from build123d import *

# Parameters (mm, degrees)
SKETCH1_R           = 50.8
BOSS_EXTRUDE1_DEPTH = 25
FILLET2_R           = 8
FILLET3_R           = 8
SKETCH2_R           = 15
BOSS_EXTRUDE2_DEPTH = 5
SKETCH3_R           = 12
CUT_EXTRUDE1_DEPTH  = 5
FILLET4_R           = 8
SKETCH5_R           = 3.165
CUT_EXTRUDE2_DEPTH  = 78.85422275
CUT_EXTRUDE3_DEPTH  = 78.85422275


with BuildPart() as part:
    # Sketch1 → Boss-Extrude1 (new body)
    with BuildSketch(Plane(origin=(0, 0, 0), x_dir=(1, 0, 0), z_dir=(0, 1, 0))):
        with Locations(Location((0, 0, 0), (0, 0, 270))):
            Circle(SKETCH1_R)
    extrude(amount=BOSS_EXTRUDE1_DEPTH)

    # Fillet2
    fillet2_edges = [part.edges().sort_by_distance(p)[0] for p in [
        (0, 25, -50.8),
    ]]
    fillet(fillet2_edges, radius=FILLET2_R)

    # Fillet3
    fillet3_edges = [part.edges().sort_by_distance(p)[0] for p in [
        (0, 0, -50.8),
    ]]
    fillet(fillet3_edges, radius=FILLET3_R)

    # Sketch2 → Boss-Extrude2 (add)
    with BuildSketch(Plane.XZ):
        with Locations(Location((0, 0, 0), (0, 0, 90))):
            Circle(SKETCH2_R)
    extrude(amount=BOSS_EXTRUDE2_DEPTH)

    # Sketch3 → Cut-Extrude1 (cut)
    with BuildSketch(Plane(origin=(0, 25, 0), x_dir=(1, 0, 0), z_dir=(0, 1, 0))):
        with Locations(Location((0, 0, 0), (0, 0, 270))):
            Circle(SKETCH3_R)
    extrude(amount=-CUT_EXTRUDE1_DEPTH, mode=Mode.SUBTRACT)

    # Fillet4
    # the kernel refuses this fillet: 8 mm, written as the material it adds along each edge
    with BuildSketch(Plane(origin=(0, 0, 0), x_dir=(0, 0, 1), z_dir=(1, 0, 0))) as fillet4_piece_1:
        with BuildLine():
            CenterArc((22.416198487, 8), FILLET4_R, 202.024312837, 67.975687163)
            Line((15, 5), (14.85167603, 4.94))
            ThreePointArc((14.85167603, 4.94), (14.84, 2.5), (14.84, 0))
            Line((14.84, 0), (15, -0.16))
            Line((15, -0.16), (22.416198487, -0.16))
            Line((22.416198487, -0.16), (22.416198487, 0))
        make_face()
    revolve(axis=Axis((0, 0, 0), (0, -1, 0)))

    # Sketch5 → Cut-Extrude2 (cut, through all)
    with BuildSketch(Plane.XZ.offset(5)):
        with Locations(Location((0, 0, 0), (0, 0, 270))):
            Circle(SKETCH5_R)
    extrude(amount=-CUT_EXTRUDE2_DEPTH, mode=Mode.SUBTRACT)

    # Sketch6 → Cut-Extrude3 (cut, through all)
    with BuildSketch(Plane(origin=(0, 25, 0), x_dir=(1, 0, 0), z_dir=(0, 1, 0))):
        with BuildLine():
            Line((6.669640143, 14.619160774), (17.119775233, 37.524775128))
            ThreePointArc((17.119775233, 37.524775128), (-2.42176691, 41.174391282), (-21.4007271, 35.259102825))
            Line((-21.4007271, 35.259102825), (-8.337442905, 13.736484528))
            ThreePointArc((-8.337442905, 13.736484528), (-0.943488661, 16.041003414), (6.669640143, 14.619160774))
        make_face()
        with BuildLine():
            Line((13.736484528, 8.337442905), (35.259102825, 21.4007271))
            ThreePointArc((35.259102825, 21.4007271), (41.174391282, 2.42176691), (37.524775128, -17.119775233))
            Line((37.524775128, -17.119775233), (14.619160774, -6.669640143))
            ThreePointArc((14.619160774, -6.669640143), (16.041003414, 0.943488661), (13.736484528, 8.337442905))
        make_face()
        with BuildLine():
            Line((8.337442905, -13.736484528), (21.4007271, -35.259102825))
            ThreePointArc((21.4007271, -35.259102825), (2.42176691, -41.174391282), (-17.119775233, -37.524775128))
            Line((-17.119775233, -37.524775128), (-6.669640143, -14.619160774))
            ThreePointArc((-6.669640143, -14.619160774), (0.943488661, -16.041003414), (8.337442905, -13.736484528))
        make_face()
        with BuildLine():
            Line((-13.736484528, -8.337442905), (-35.259102825, -21.4007271))
            ThreePointArc((-35.259102825, -21.4007271), (-41.174391282, -2.42176691), (-37.524775128, 17.119775233))
            Line((-37.524775128, 17.119775233), (-14.619160774, 6.669640143))
            ThreePointArc((-14.619160774, 6.669640143), (-16.041003414, -0.943488661), (-13.736484528, -8.337442905))
        make_face()
    extrude(amount=-CUT_EXTRUDE3_DEPTH, mode=Mode.SUBTRACT)


solid = part.part
The listing builds one solid part. Answer for the finished solid, in the listing's coordinates (mm). A direction names the side the tool comes from. Coordinates: 2 decimals unless noted, no trailing zeros. Write each loop counter-clockwise with the first axis right and the second up, starting at its lowest first coordinate (ties: lowest second). Pieces come first, ordered by that corner, then holes. Notation, with made-up numbers: (15.25, 6.25) - (45.25, 6.25) arc R11 cw to (45.25, 10.25) - close; hole circle Ø9 at (42.25, -5). An arc over 180 degrees is marked (long way). Answer as CSV lines item,"result".
1. Find section D-D (y = -1.5). Give the vertices of the cut face in (x, z) (1 decimal).
Computed values:
outline,"(-16.2, -7.4) arc R17.8 ccw to (-9.2, -15.2) - (-8.3, -13.7) arc R16.1 ccw to (6.7, -14.6) - (7.4, -16.2) arc R17.8 ccw to (15.2, -9.2) - (13.7, -8.3) arc R16.1 ccw to (14.6, 6.7) - (16.2, 7.4) arc R17.8 ccw to (9.2, 15.2) - (8.3, 13.7) arc R16.1 ccw to (-6.7, 14.6) - (-7.4, 16.2) arc R17.8 ccw to (-15.2, 9.2) - (-13.7, 8.3) arc R16.1 ccw to (-14.6, -6.7) - close; hole circle Ø6.3 at (0, 0)"
2. Straight lines are drawn through the part: line 1 (X direction, y = 9.75, z = 0) (3 decimals); line 2 (X direction, y = 16, z = 5); line 3 (Z direction, x = 11, y = 17.5). For each, find the intervals that lie inside material, in ascending order. Write a range as [from, to].
Computed values:
line 1,"x = [-50.8, -41.246], [-16.069, -3.165], [3.165, 16.069], [41.246, 50.8]"
line 2,"x = [-50.55, -40.94], [-15.27, 15.27], [40.94, 50.55]"
line 3,"z = [-49.58, -39.75], [-24.11, 18.12], [39.75, 49.58]"
3. Find section B-B (z = 0). Give the vertices of the cut face in (x, y) (3 decimals), plus the area to 3 significant figures.
Computed values:
outline,"(-50.8, 8) arc R8 ccw to (-42.8, 0) - (-41.246, 0) - (-41.246, 25) - (-42.8, 25) arc R8 ccw to (-50.8, 17) - close; (-16.069, -3.131) arc R8 cw to (-15, -5) - (-3.165, -5) - (-3.165, 20) - (-12, 20) - (-12, 25) - (-16.069, 25) - close; (3.165, -5) - (15, -5) arc R8 cw to (16.069, -3.131) - (16.069, 25) - (12, 25) - (12, 20) - (3.165, 20) - close; (41.246, 0) - (42.8, 0) arc R8 ccw to (50.8, 8) - (50.8, 17) arc R8 ccw to (42.8, 25) - (41.246, 25) - close"
area,"1,110 mm²"
4. Determine the mould class of faces 1 (the flat face through (-26.232, 11.132, -11.968)), 2 (the cylindrical face through (-30.911, 12.437, -40.313)), 3 (the flat face through (-12.5, 25, -0.2)) for opening direction Z: +Z half, -Z half, draft (parallel to the pull), parting line (faces both ways), or undercut.
Computed values:
face 1,"undercut"
face 2,"parting line"
face 3,"draft"
5. Given P1, Ø5, axis at x = -15, z = 9.5, coming from the -Y side; P2, Ø7, axis at x = -2, z = -1, coming from the +Y side; P3, Ø2, axis at y = 7.5, z = 32, coming from the +X side, each flat-ended and moving along its own axis, determine where each tip first touches the part or whether it passes through.
Computed values:
P1,"stops at y = -4.43"
P2,"stops at y = 20"
P3,"stops at x = 40.23"
6. Find section C-C (y = 5.5). Give the vertices of the cut face in (x, z) (3 decimals).
Computed values:
outline,"circle Ø100.799 at (0, 0); hole (-37.525, -17.12) - (-14.619, -6.67) arc R16.069 cw to (-13.736, 8.337) - (-35.259, 21.401) arc R41.246 ccw to start; hole (-21.401, -35.259) arc R41.246 ccw to (17.12, -37.525) - (6.67, -14.619) arc R16.069 cw to (-8.337, -13.736) - close; hole (-17.12, 37.525) - (-6.67, 14.619) arc R16.069 cw to (8.337, 13.736) - (21.401, 35.259) arc R41.246 ccw to start; hole circle Ø6.33 at (0, 0); hole (13.736, -8.337) - (35.259, -21.401) arc R41.246 ccw to (37.525, 17.12) - (14.619, 6.67) arc R16.069 cw to start"
7. A tool of negligible diameter and unlimited length cuts with its end or side. For faces 4 (the flat face through (-4, -5, 0)), 5 (the flat face through (-19, 0, -13)), 6 (the cylindrical face through (-16.047, 11.132, 0.834)), 7 (the flat face through (-2.5, 20, 2.5)), from which of +Z, -Z, +X, -X, +Y, -Y can it reach the whole face along a straight path? Write none if from no direction.
Computed values:
face 4,"+Z, -Z, +X, -X, -Y"
face 5,"-Y"
face 6,"+Y, -Y"
face 7,"+Y"
8. Find section A-A (x = 0). Give the vertices of the cut face in (y, z) (3 decimals).
Computed values:
outline,"(-5, -15) arc R8 cw to (-3.131, -16.069) - (25, -16.069) - (25, -12) - (20, -12) - (20, -3.165) - (-5, -3.165) - close; (-5, 3.165) - (20, 3.165) - (20, 12) - (25, 12) - (25, 16.069) - (-3.131, 16.069) arc R8 cw to (-5, 15) - close; (0, -42.8) arc R8 ccw to (8, -50.8) - (17, -50.8) arc R8 ccw to (25, -42.8) - (25, -41.246) - (0, -41.246) - close; (0, 41.246) - (25, 41.246) - (25, 42.8) arc R8 ccw to (17, 50.8) - (8, 50.8) arc R8 ccw to (0, 42.8) - close"
